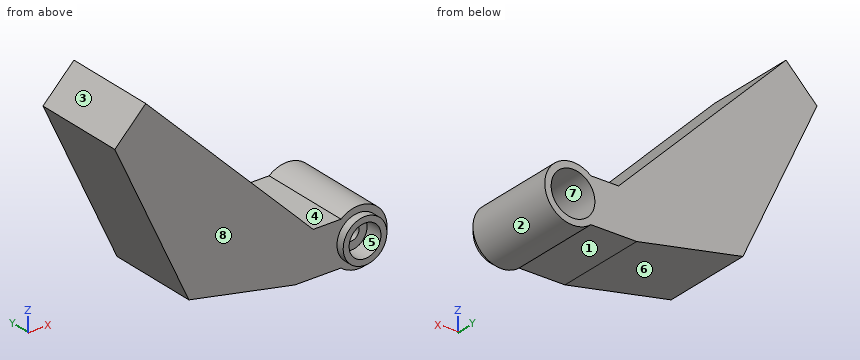
from build123d import *

# Parameters (mm, degrees)
SKETCH1_R            = 3.43
SKETCH1_R_2          = 1.235
MAIN_BODY_DEPTH      = 4.715
SKETCH2_R            = 2.45
TOP_SCREW_HOLE_DEPTH = 0.865
MAKE_START           = -3.465
MAKE_WINGS_DEPTH     = 14.465
SKETCH4_R            = 2.5
SPLINE_HOLE_DEPTH    = 2.8
SKETCH5_W            = 6.86
SKETCH5_H            = 14.465
BOSS_EXTRUDE1_DEPTH  = 5
BOSS_EXTRUDE2_DEPTH  = 14.465
BOSS_EXTRUDE3_DEPTH  = 14.465
BOSS_EXTRUDE4_START  = -14.465
BOSS_EXTRUDE4_DEPTH  = 14.465
CUT_EXTRUDE1_DEPTH   = 51.941486893


with BuildPart() as part:
    # Sketch1 → main body (new body)
    with BuildSketch(Plane(origin=(0, 0, 0), x_dir=(1, 0, 0), z_dir=(0, 1, 0))):
        with Locations(Location((0, 0, 0), (0, 0, 90))):
            Circle(SKETCH1_R)
        with Locations(Location((0, 0, 0), (0, 0, 90))):
            Circle(SKETCH1_R_2, mode=Mode.SUBTRACT)
    extrude(amount=MAIN_BODY_DEPTH)

    # Sketch2 → top screw hole (cut)
    with BuildSketch(Plane(origin=(0, 4.715, 0), x_dir=(1, 0, 0), z_dir=(0, 1, 0))):
        with Locations(Location((0, 0, 0), (0, 0, 270))):
            Circle(SKETCH2_R)
    extrude(amount=-TOP_SCREW_HOLE_DEPTH, mode=Mode.SUBTRACT)

    # Sketch3 → make wings (add)
    with BuildSketch(Plane(origin=(0, 4.715, 0), x_dir=(1, 0, 0), z_dir=(0, 1, 0)).offset(MAKE_START)):
        with BuildLine():
            ThreePointArc((0, -3.43), (-3.43, 0), (0, 3.43))
            Line((0, 3.43), (-6.57, 3.43))
            ThreePointArc((-6.57, 3.43), (-10, 0), (-6.57, -3.43))
            Line((-6.57, -3.43), (0, -3.43))
        make_face()
    extrude(amount=MAKE_WINGS_DEPTH)

    # Sketch4 → spline hole (cut)
    with BuildSketch(Plane.XZ):
        with Locations(Location((0, 0, 0), (0, 0, 270))):
            Circle(SKETCH4_R)
    extrude(amount=-SPLINE_HOLE_DEPTH, mode=Mode.SUBTRACT)

    # Sketch5 → Boss-Extrude1 (add)
    with BuildSketch(Plane.ZY.offset(10)):
        with Locations((0, 8.4825)):
            Rectangle(SKETCH5_W, SKETCH5_H)
    extrude(amount=-BOSS_EXTRUDE1_DEPTH)

    # Sketch6 → Boss-Extrude2 (add)
    with BuildSketch(Plane(origin=(0, 15.715, 0), x_dir=(1, 0, 0), z_dir=(0, 1, 0))):
        Polygon((-10, 3.43), (-38.284271247, -24.854271247), (-33.433518729, -29.705023766), (-5.149247481, -1.420752519), align=None)
    extrude(amount=-BOSS_EXTRUDE2_DEPTH)

    # Sketch7 → Boss-Extrude3 (add)
    with BuildSketch(Plane(origin=(0, 15.715, 0), x_dir=(1, 0, 0), z_dir=(0, 1, 0))):
        Polygon((-38.284271247, -24.854271247), (-20.294632832, 13.724632832), (-10, 3.43), align=None)
    extrude(amount=-BOSS_EXTRUDE3_DEPTH)

    # Sketch9 → Boss-Extrude4 (add)
    with BuildSketch(Plane(origin=(0, 15.715, 0), x_dir=(1, 0, 0), z_dir=(0, 1, 0)).offset(BOSS_EXTRUDE4_START)):
        with BuildLine():
            Line((0, 3.43), (-2.803569154, 3.43))
            ThreePointArc((-2.803569154, 3.43), (4.43, 0), (-2.803569154, -3.43))
            Line((-2.803569154, -3.43), (0, -3.43))
            ThreePointArc((0, -3.43), (3.43, 0), (0, 3.43))
        make_face()
    extrude(amount=BOSS_EXTRUDE4_DEPTH)

    # Sketch10 → Cut-Extrude1 (cut, through all)
    with BuildSketch(Plane(origin=(0, 15.715, 0), x_dir=(1, 0, 0), z_dir=(0, 1, 0))):
        Polygon((-10, 3.43), (-26.663813955, 0.065879836), (-20.294632832, 13.724632832), align=None)
    extrude(amount=-CUT_EXTRUDE1_DEPTH, mode=Mode.SUBTRACT)


solid = part.part
Can you work these out from the model? Positions are in its coordinate system, mm. Face numbers are marked on the shaded views. A direction names the side the tool comes from. Coordinates: 2 decimals unless noted, no trailing zeros. Loops run counter-clockwise (first coordinate to the right, second up) from the corner with the lowest first, then second, coordinate; pieces in that order, holes last. Notation, with made-up numbers: M 72.25,47 L 113.25,47 A18 ccw 113.25,62 Z; hole C 79,62.25 d10. An arc over 180 degrees is marked long. Return JSON: item names as keys, results as strings. Group by question number.
Item 1: If I drill on L1, parallel to Y at x = -24, z = 19 (3 decimals); L2, parallel to X at y = 8.5, z = 0; L3, parallel to Z at x = -6, y = 13.25, over which ranges is the centre line in solid material (lowest first)? Write a range as from..to.
Item 2: On a 3-axis mill with a long thin cutter (end or side, diameter ignored), from which of +Z, -Z, +X, -X, +Y, -Y can I reach the whole of each face in a straight line? I mean the marked faces 1, 2, 3, 4 and 5. Say none if no direction works.
Item 3: I'm going to push flat-ended pins straight in: pin 1 Ø6 at (y, z) = (4.5, 14) entering from -X; pin 2 Ø3 at (x, z) = (0, 0) entering from -Y; pin 3 Ø1 at (x, y) = (-24, 14) entering from +Z. Where does each tip first touch, or does it pass through?
Item 4: Imagine slicing it at B-B (y = 6.5). Please give me the cut outline in (x, z), and give its area (3 significant figures).
Item 5: Thinking about a two-plate mould opening in X: for the marked faces 6, 7 and 8, which applies, released by +X, released by -X, zero draft, split by the parting line, or undercut?
Item 6: Imagine slicing it at A-A (x = 0). Please give me the cut outline in (y, z) (3 decimals).
Verdict:
{
 "1": {"L1": "y = 1.25..15.715", "L2": "x = -26.69..-3.43, 3.43..4.43", "L3": "z = -3.43..3.43"},
 "2": {"face 1": "-Z, -X, +Y, -Y", "face 2": "+Y, -Y", "face 3": "+Z, -X, +Y, -Y", "face 4": "+Z, +Y, -Y", "face 5": "-Y"},
 "3": {"pin 1": "stops at x = -34.62", "pin 2": "stops at y = 2.8", "pin 3": "stops at z = 20.77"},
 "4": {"outline": "M -38.28,24.85 L -26.66,-0.07 L -10,-3.43 L -2.8,-3.43 A4.43 ccw long -2.8,3.43 L -7.16,3.43 L -33.43,29.71 Z; hole C 0,0 d6.86", "area": "509 mm^2"},
 "5": {"face 6": "released by -X", "face 7": "undercut", "face 8": "zero draft"},
 "6": {"outline": "M 0,-3.43 L 1.25,-3.43 L 1.25,-4.43 L 15.715,-4.43 L 15.715,-3.43 L 4.715,-3.43 L 4.715,-2.45 L 3.85,-2.45 L 3.85,-1.235 L 2.8,-1.235 L 2.8,-2.5 L 0,-2.5 Z; M 0,2.5 L 2.8,2.5 L 2.8,1.235 L 3.85,1.235 L 3.85,2.45 L 4.715,2.45 L 4.715,3.43 L 15.715,3.43 L 15.715,4.43 L 1.25,4.43 L 1.25,3.43 L 0,3.43 Z"}
}
